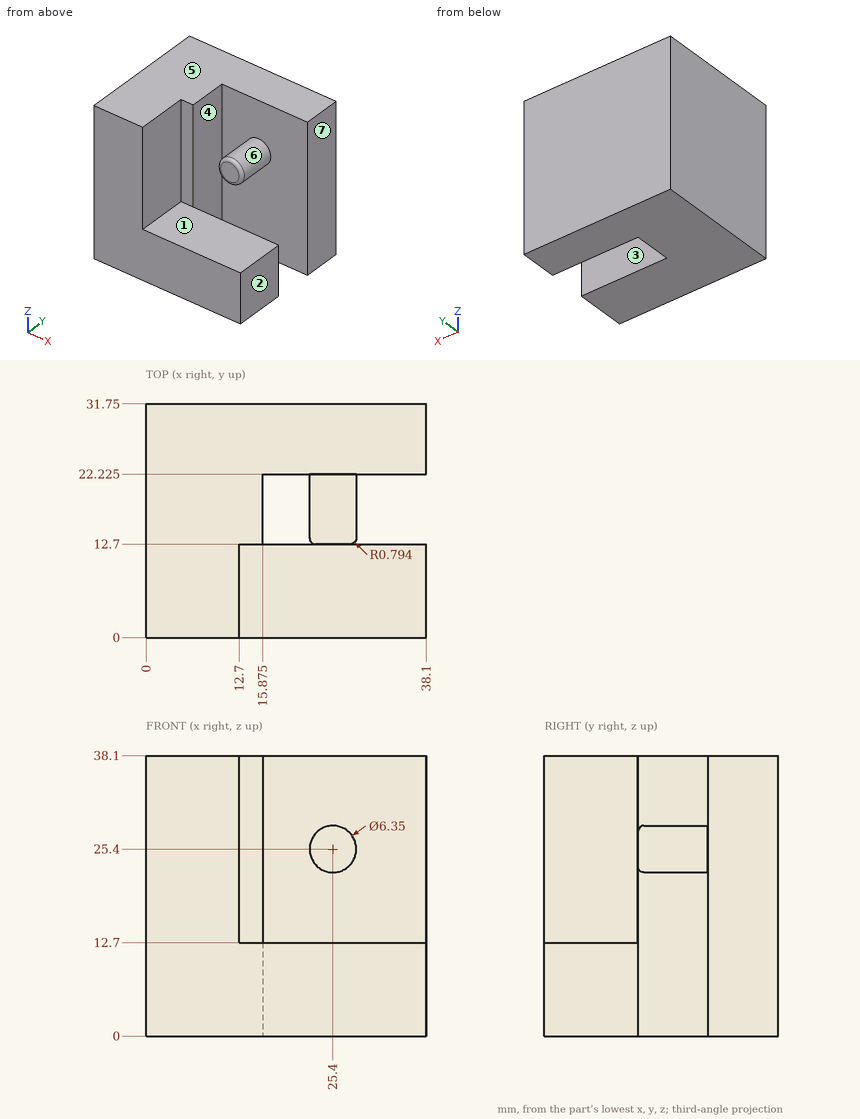
Source: three-view drawing plus pictorial views. Frame: mm from the lowest corner of the part. A direction names the side the tool comes from. Give positions to 0.01 mm unless a question says otherwise; leave off trailing zeros. Put each result on its own line as item: value.
Q1. Reachability of the marked faces 1, 2, 3 and 4 from +Z, -Z, +X, -X, +Y, -Y: full face, straight path, thin tool, end or side. Return the list, or none.
Here are the results:
face 1: +Z, +X, -Y
face 2: +Z, -Z, +X, +Y, -Y
face 3: -Z, +X
face 4: +Z, -Z
Q2. Material intervals for L1, parallel to X at y = 7, z = 35.5; L2, parallel to Y at x = 23.5, z = 25; L3, parallel to X at y = 18.5, z = 20 (1 decimal), sorted ascending.
Here are the results:
L1: x = 0 to 12.7
L2: y = 12.7 to 31.75
L3: x = 0 to 15.9
Q3. Pin query (flat end, axial travel): pin 1 (5 mm diameter, centred on x = 25, z = 26.5, fed in from -Y); pin 2 (14 mm diameter, centred on x = 26, y = 8.5, fed in from +Z) (3 decimals); pin 3 (6.5 mm diameter, centred on y = 6.5, z = 30, fed in from +X). Return the tip coordinate at first contact, or that it passes through.
Here are the results:
pin 1: stops at y = 12.7
pin 2: stops at z = 28.575
pin 3: stops at x = 12.7
Q4. Draft query along X for the marked faces 5, 6 and 7. Return one class per face: released by +X, released by -X, zero draft, split by the parting line, or undercut.
Here are the results:
face 5: zero draft
face 6: undercut
face 7: released by +X
